Geometry: final body of the model. Coordinates: model frame, mm. A direction names the side the tool comes from. Give positions to 0.01 mm unless a question says otherwise; leave off trailing zeros. Write each loop counter-clockwise with the first axis right and the second up, starting at its lowest first coordinate (ties: lowest second). Pieces come first, ordered by that corner, then holes. Notation, with made-up numbers: M -8,42.25 L 26,42.25 A28 ccw 26,73.25 Z; hole C 61,88.25 d1. An arc over 180 degrees is marked long. Answer as a JSON object with one key per item and string values.
from build123d import *

# Parameters (mm, degrees)
F1_DEPTH = 30
F2_T     = -2
F3_R     = 5
F4_R     = 4
F5_DEPTH = 2.001
F6_R     = 4
F7_DEPTH = 2.001


with BuildPart() as f1:
    # F0 (on Right) → F1 (new body)
    with BuildSketch(Plane.YZ):
        Polygon((0, 30), (0, 0), (30, 30), align=None)
    extrude(amount=F1_DEPTH)

    # F2
    f2_openings = [f1.faces().sort_by_distance(p)[0] for p in [
        (15, 15, 15),
    ]]
    offset(amount=F2_T, openings=f2_openings)

    # F3
    f3_edges = [f1.edges().sort_by_distance(p)[0] for p in [
        (30, 0, 15),
        (30, 15, 30),
        (0, 0, 15),
        (0, 15, 30),
    ]]
    fillet(f3_edges, radius=F3_R)

    # F4 (on face) → F5 (cut, through all)
    with BuildSketch(Plane(origin=(0, 0, 28), x_dir=(1, 0, 0), z_dir=(0, 0, -1))):
        with Locations((15, -15)):
            Circle(F4_R)
    extrude(amount=-F5_DEPTH, mode=Mode.SUBTRACT)

    # F6 (on face) → F7 (cut, through all)
    with BuildSketch(Plane(origin=(0, 2, 0), x_dir=(-1, 0, 0), z_dir=(0, 1, 0))):
        with Locations((-15, 15)):
            Circle(F6_R)
    extrude(amount=-F7_DEPTH, mode=Mode.SUBTRACT)


solid = f1.part
1) Set-up query: faces 1 (the flat face through (28, 12, 18)), 2 (the flat face through (0, 13, 17)). Return all of +Z, -Z, +X, -X, +Y, -Y with unobstructed straight access to the full face (end or side cutting, diameter ignored); none if empty.
Geometry check:
{"face 1": "-Z, +Y", "face 2": "+Z, -Z, -X, +Y, -Y"}
2) Pull-direction query (Z, two-part tool) for faces 3 (the flat face through (12, 2, 18)), 4 (the cylindrical face through (17.95, 1.01, 17.7)), 5 (the flat face through (1, 15, 15)); classes: pulls with the +Z half, pulls with the -Z half, needs draft (parallel to the pull), parting line crosses it, or undercut.
Geometry check:
{"face 3": "needs draft", "face 4": "undercut", "face 5": "pulls with the -Z half"}
3) Cut plane B-B on x = 15. Return loops of the section in (y, z).
Geometry check:
{"outline": "M 0,0 L 2,2 L 2,11 L 0,11 Z; M 0,19 L 2,19 L 2,28 L 11,28 L 11,30 L 0,30 Z; M 19,28 L 28,28 L 30,30 L 19,30 Z"}
4) Cut plane A-A on y = 15. Return loops of the section in (x, z).
Geometry check:
{"outline": "M 0,15 L 2,15 L 2,28 L 11,28 L 11,30 L 5,30 A5 ccw 0,25 Z; M 19,28 L 28,28 L 28,15 L 30,15 L 30,25 A5 ccw 25,30 L 19,30 Z"}
5) Cut plane D-D on y = 24.5. Return loops of the section in (x, z).
Geometry check:
{"outline": "M 0,24.5 L 2,24.5 L 2,28 L 28,28 L 28,24.5 L 30,24.5 L 30,25 A5 ccw 25,30 L 5,30 A5 ccw 0,25 Z"}
6) Contact query for flat-ended pins moving along their axis: P1, Ø8, axis at x = 21.5, y = 21.5, coming from the -Z side; P2, Ø12, axis at x = 12, y = 17, coming from the +Z side; P3, Ø10.5, axis at x = 15, z = 15, coming from the +Y side. Output: stop coordinate, or through.
Geometry check:
{"P1": "stops at z = 28", "P2": "stops at z = 30", "P3": "stops at y = 2"}
7) Line query: line 1 (X direction, y = 6.5, z = 19); line 2 (Y direction, x = 19, z = 10); line 3 (Z direction, x = 16.5, y = 24). Output: solid intervals per line, ascending. Write a range as from..to.
Geometry check:
{"line 1": "x = 0..2, 28..30", "line 2": "y = 0..2", "line 3": "z = 28..30"}
8) Cut plane C-C on z = 15. Return loops of the section in (x, y).
Geometry check:
{"outline": "M 0,5 A5 ccw 5,0 L 11,0 L 11,2 L 2,2 L 2,15 L 0,15 Z; M 19,0 L 25,0 A5 ccw 30,5 L 30,15 L 28,15 L 28,2 L 19,2 Z"}
